Check sheet for the modelled part. Datum: model origin and axes. Units: mm. A direction names the side the tool comes from. Round coordinates to 2 decimals unless told otherwise and drop trailing zeros. Order: outer loops, then holes, each group sorted by start corner. A loop starts at its lowest first (then second) coordinate and runs counter-clockwise, first axis right, second up. Notation, with made-up numbers: (67, 4.5) -> (104, 4.5) arc R15 cw to (104, 18.5) -> close; hole circle Ø11 at (50.25, 48). An arc over 180 degrees is marked (long way). Answer in a Markdown table with one row per item.
from build123d import *

# Parameters (mm, degrees)
F1_DEPTH = 7
F2_R     = 10
F5_DEPTH = 4


with BuildPart() as f1:
    # F0 (on Top) → F1 (new body)
    with BuildSketch(Plane.XY):
        Polygon((-27, -20), (27, -20), (27, 20), (10, 20), (10, 40), (-10, 40), (-10, 20), (-27, 20), align=None)
    extrude(amount=F1_DEPTH)

    # F2
    f2_edges = [f1.edges().sort_by_distance(p)[0] for p in [
        (10, 20, 3.5),
        (-10, 20, 3.5),
    ]]
    fillet(f2_edges, radius=F2_R)

    # F4 (on offset) → F5 (join)
    with BuildSketch(Plane.YZ.offset(23)):
        with BuildLine():
            Line((-19.987991, 7), (20, 7))
            Line((20, 7), (20, 25.208094))
            ThreePointArc((20, 25.208094), (19.774022, 26.131591), (19.147153, 26.846398))
            Line((19.147153, 26.846398), (4.845687, 36.860392))
            ThreePointArc((4.845687, 36.860392), (4.22884, 37.828648), (4.477324, 38.949485))
            Line((4.477324, 38.949485), (37.542201, 86.171024))
            ThreePointArc((37.542201, 86.171024), (37.421504, 87.69386), (35.903428, 87.864272))
            ThreePointArc((35.903428, 87.864272), (0.076045, 53.010837), (-19.952304, 7.215329))
            ThreePointArc((-19.952304, 7.215329), (-19.973087, 7.108152), (-19.987991, 7))
        make_face()
    extrude(amount=F5_DEPTH)


solid = f1.part
Item 1: Cross-section at D-D (y = -8). Record the boundary of the cut face in (x, z), and give its area (3 significant figures).
Result sheet:
| item | result |
|---|---|
| outline | (-27, 0) -> (27, 0) -> (27, 39.72) -> (23, 39.72) -> (23, 7) -> (-27, 7) -> close |
| area | 509 mm^2 |
Item 2: Depth check by flat-ended pin: P1, Ø3, axis at x = 17, y = 12.5, coming from the +Z side; P2, Ø17.5, axis at y = 11, z = 51, coming from the -X side; P3, Ø5.5, axis at y = 33, z = 4, coming from the -X side. Enter the tip coordinate at first touch or a pass-through.
Result sheet:
| item | result |
|---|---|
| P1 | stops at z = 7 |
| P2 | stops at x = 23 |
| P3 | stops at x = -10 |
Item 3: Cross-section at C-C (z = 12.5). Record the boundary of the cut face in (x, y).
Result sheet:
| item | result |
|---|---|
| outline | (23, -18.66) -> (27, -18.66) -> (27, 20) -> (23, 20) -> close |
Item 4: Mould release check, pull along Z, two halves, no side actions. Record for faces 4 (the flat face through (0, 4, 0)), 5 (the flat face through (10, 35, 3)), 6 (the flat face through (24.97, 12.1, 31.78)): pulls with the +Z half, pulls with the -Z half, needs draft (parallel to the pull), parting line crosses it, or undercut.
Result sheet:
| item | result |
|---|---|
| face 4 | pulls with the -Z half |
| face 5 | needs draft |
| face 6 | undercut |
Item 5: Set-up check for faces 1 (the flat face through (-10, 35, 3)), 2 (the flat face through (24.97, 20.78, 62.23)), 3 (the flat face through (24, 20, 10)): record each of +Z, -Z, +X, -X, +Y, -Y from which the full face is reachable in a straight line by a thin tool's end or side.
Result sheet:
| item | result |
|---|---|
| face 1 | +Z, -Z, -X, +Y |
| face 2 | +X, -X, +Y |
| face 3 | -Z, +X, +Y |
Item 6: Cross-section at B-B (x = -8.5). Record the boundary of the cut face in (y, z).
Result sheet:
| item | result |
|---|---|
| outline | (-20, 0) -> (40, 0) -> (40, 7) -> (-20, 7) -> close |
Item 7: Scan lines: line 1 (Z direction, x = 4.5, y = 26); line 2 (X direction, y = 11, z = 56); line 3 (Z direction, x = 24, y = -1.5). Record each from-to range of solid material in increasing order. Write a range as [from, to].
Result sheet:
| item | result |
|---|---|
| line 1 | z = [0, 7] |
| line 2 | x = [23, 27] |
| line 3 | z = [0, 50.68] |
Item 8: Cross-section at A-A (y = 12). Record the boundary of the cut face in (x, z).
Result sheet:
| item | result |
|---|---|
| outline | (-27, 0) -> (27, 0) -> (27, 31.85) -> (23, 31.85) -> (23, 7) -> (-27, 7) -> close; (23, 49.69) -> (27, 49.69) -> (27, 67.79) -> (23, 67.79) -> close |
